Verification items for this drawing (mm, ordinates from the low corner). A direction names the side the tool comes from. Coordinates: 2 decimals unless noted, no trailing zeros. Loops run counter-clockwise (first coordinate to the right, second up) from the corner with the lowest first, then second, coordinate; pieces in that order, holes last. Notation, with made-up numbers: (54.5, 84) - (68.5, 84) arc R32 cw to (68.5, 120) - close; hole circle Ø7 at (78, 56.5). An arc over 180 degrees is marked (long way). One line per item, written item: value. Start each with the question number.
(1) Set-up check for the marked faces 4, 5 and 6: record each of +Z, -Z, +X, -X, +Y, -Y from which the full face is reachable in a straight line by a thin tool's end or side.
(2) Section check D-D (x = 0.9). Record the boundary of the cut face in (y, z), plus the area to 3 significant figures.
(3) Thickness scan on probe 1 along X at (y, z) = (2.95, 0.25); probe 2 along Y at (x, z) = (2.2, 1.15); probe 3 along X at (y, z) = (3.7, 3.85). Record the ranges inside material, lowest first. Write a range as [from, to].
(4) Gauge pin test, flat ends, axial feed: P1, Ø0.9, axis at y = 1, z = 2.5, coming from the -X side; P2, Ø0.8, axis at x = 0.5, z = 3.5, coming from the -Y side. Record the tip position at first contact, or that the pin passes through.
(5) Section check B-B (z = 0.9). Record the boundary of the cut face in (x, y), plus the area to 3 significant figures.
(6) Section check C-C (y = 2.5). Record the boundary of the cut face in (x, z), plus the area to 3 significant figures.
(7) Draft check along Z on the marked faces 1, 2 and 3. Enter one of: +Z half, -Z half, draft (parallel to the pull), parting line (faces both ways), or undercut.
(8) Section check A-A (x = 2.1). Record the boundary of the cut face in (y, z).
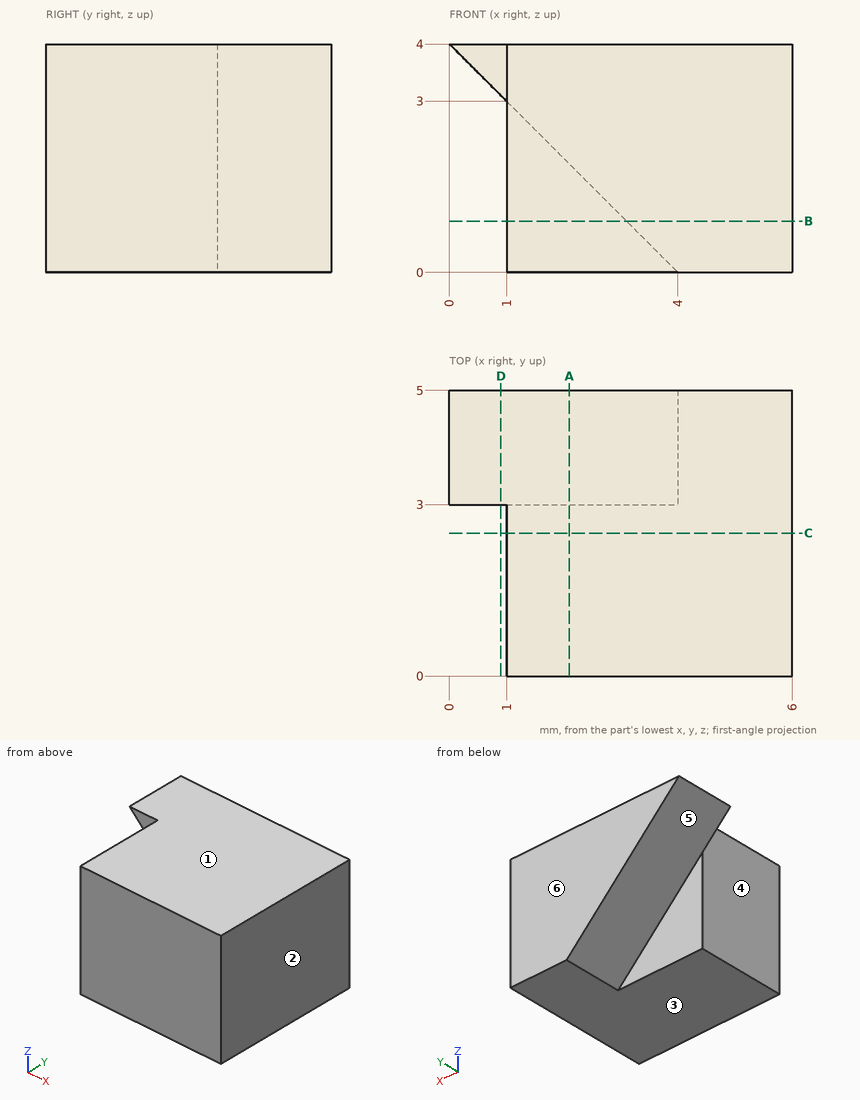
Responses:
1. face 4: +Z, -Z, -X, -Y
1. face 5: -Z, -X, +Y
1. face 6: +Z, -Z, +X, -X, +Y
2. outline: (3, 3.1) - (5, 3.1) - (5, 4) - (3, 4) - close
2. area: 1.80 mm²
3. probe 1: x = [1, 6]
3. probe 2: y = [0, 3]
3. probe 3: x = [0.15, 6]
4. P1: stops at x = 1
4. P2: stops at y = 3
5. outline: (1, 0) - (6, 0) - (6, 5) - (3.1, 5) - (3.1, 3) - (1, 3) - close
5. area: 20.8 mm²
6. outline: (1, 0) - (6, 0) - (6, 4) - (1, 4) - close
6. area: 20.0 mm²
7. face 1: +Z half
7. face 2: draft
7. face 3: -Z half
8. outline: (0, 0) - (3, 0) - (3, 1.9) - (5, 1.9) - (5, 4) - (0, 4) - close
